For this review, take the finished solid that the model builds, in its own axes (mm). A direction names the side the tool comes from. Coordinates: 2 decimals unless noted, no trailing zeros. Write each loop counter-clockwise with the first axis right and the second up, starting at its lowest first coordinate (ties: lowest second). Pieces come first, ordered by that corner, then holes.
1) We need section B-B on z = -33.25. Write out the cut boundary in (x, y).
2) Insertion check: P1, Ø10, axis at x = 11.5, y = -4.5, coming from the -Z side (3 decimals); P2, Ø10.5, axis at x = 19.5, y = -7.5, coming from the -Z side; P3, Ø6.5, axis at x = 25.84, z = -39.9, coming from the -Y side. Each pin has a flat end and moves straight along its axis. Give the tip position at first contact, or say it passes through.
3) For faces 4 (the face through (30.226, 4.09, -39.007)), 5 (the face through (25, 5.076, -30)), 6 (the face through (31.338, -19, -34)), 7 (the face through (26, -7, -29.903)), 8 (the face through (30.487, -12.894, -27.438)), list the 3-axis set-ups (+Z, -Z, +X, -X, +Y, -Y) from which the entire face can be reached by the end or side of a thin tool; tool diameter is ignored.
4) To check wall thickness, follow line 1 along X through (y, z) = (-13, -28); line 2 along Y through (x, z) = (48.5, -32.5); line 3 along Y through (x, z) = (42, -28.25). State the ranges of each line that lie inside material, in increasing order.
5) We need section D-D on y = 1.75. Write out the cut boundary in (x, z).
6) We need section A-A on x = 44.5. Write out the cut boundary in (y, z).
7) Mouldability with a two-part tool opening along X and no side actions: class faces 1 (the face through (25.911, 4.09, -43.903)), 2 (the face through (49, -8, -34.903)), 3 (the face through (30.487, 1.906, -27.438)) as pulls with the +X half, pulls with the -X half, needs draft (parallel to the pull), parting line crosses it, or undercut.
8) We need section C-C on y = -13.5. Write out the cut boundary in (x, z), then the cut area to 3 significant figures.
Autodesk Inventor part; units mm, degrees
ref_plane "Plano de trabalho1" through (25.8382, -7.4236, -29.9034) normal (0, 0, 1) x (1, 0, 0)
ref_plane "Plano de trabalho2" through (25.638, 5.0764, -94.896) normal (0, -1, 0) x (0, 0, 1)
ref_plane "YZ Plane" through (0, 0, 0) normal (1, 0, 0) x (0, 1, 0)
ref_plane "Plano de trabalho1" through (25.8382, -7.4236, -29.9034) normal (0, 0, 1) x (1, 0, 0)
sketch "Esboço1" plane through (25.8382, -7.4236, -29.9034) normal (0, 0, 1) x (1, 0, 0)
  line L0 (-23, 10.5) -> (23, 10.5)
  line L1 (23, 10.5) -> (23, -10.5)
  line L2 (23, -10.5) -> (-23, -10.5)
  line L3 (-23, -10.5) -> (-23, 10.5)
  line L4 (23, 12.5) -> (-23, 12.5)
  line L5 (-25, 10.5) -> (-25, -10.5)
  line L6 (-23, -12.5) -> (23, -12.5)
  line L7 (25, -10.5) -> (25, 10.5)
  arc A0 (23, -12.5) -> (25, -10.5) centre (23, -10.5) ccw
  arc A1 (-25, -10.5) -> (-23, -12.5) centre (-23, -10.5) ccw
  circle A2 centre (-13, 0) radius 8.5
  circle A3 centre (13, 0) radius 8.5
  line L8 (-23, 10.5) -> (23, -10.5) construction
  line L9 (23, 10.5) -> (-23, -10.5) construction
  line L10 (-3.25, 4.9) -> (3.25, 4.9)
  line L11 (5.25, 6.9) -> (5.25, 7.9)
  line L12 (3.25, 9.9) -> (-3.25, 9.9)
  line L13 (-5.25, 7.9) -> (-5.25, 6.9)
  line L14 (-5.25, 4.9) -> (5.25, 9.9) construction
  line L15 (5.25, 4.9) -> (-5.25, 9.9) construction
  arc A4 (-3.25, 9.9) -> (-5.25, 7.9) centre (-3.25, 7.9) ccw
  arc A5 (-5.25, 6.9) -> (-3.25, 4.9) centre (-3.25, 6.9) ccw
  arc A6 (3.25, 4.9) -> (5.25, 6.9) centre (3.25, 6.9) ccw
  arc A7 (5.25, 7.9) -> (3.25, 9.9) centre (3.25, 7.9) ccw
  line L16 (0, 0) -> (0, -7.4)
  line L17 (-3.25, -9.9) -> (3.25, -9.9)
  line L18 (5.25, -7.9) -> (5.25, -6.9)
  line L19 (3.25, -4.9) -> (-3.25, -4.9)
  line L20 (-5.25, -6.9) -> (-5.25, -7.9)
  line L21 (-5.25, -9.9) -> (5.25, -4.9) construction
  line L22 (5.25, -9.9) -> (-5.25, -4.9) construction
  arc A8 (-3.25, -4.9) -> (-5.25, -6.9) centre (-3.25, -6.9) ccw
  arc A9 (-5.25, -7.9) -> (-3.25, -9.9) centre (-3.25, -7.9) ccw
  arc A10 (3.25, -9.9) -> (5.25, -7.9) centre (3.25, -7.9) ccw
  arc A11 (5.25, -6.9) -> (3.25, -4.9) centre (3.25, -6.9) ccw
  line L23 (-23, 12.5) -> (-25, 12.5)
  line L24 (-25, 12.5) -> (-25, 10.5)
  line L25 (23, 12.5) -> (25, 12.5)
  line L26 (25, 12.5) -> (25, 10.5)
  point P0 (-25.8382, 7.4236)
  dimension "d0" = 2
  dimension "d4" = 46
  dimension "d5" = 21
  dimension "d7" = 17
  dimension "d9" = 17
  dimension "d16" = 7.4
extrude "Extrusão1" add sketch "Esboço1" along normal blind 5 contours L0 L1 L2 L3 | L25 L26 L7 A0 L6 A1 L5 L24 L23 L4
extrude "Extrusão2" add sketch "Esboço1" against normal blind 5 contours L25 L26 L7 A0 L6 A1 L5 L24 L23 L4
sketch "Esboço2" plane through (2.8382, -19.9236, -24.9034) normal (0, -1, 0) x (1, 0, 0)
  line L0 (28.5, -9.5) -> (28.5, -7.75)
  line L1 (28.5, -7.75) -> (17.5, -7.75)
  line L2 (17.5, -7.75) -> (17.5, -9.5)
  line L3 (46, -10) -> (0, -10)
  line L4 (17.5, -10) -> (28.5, -10)
  line L5 (23, -12) -> (31, -12)
  line L6 (23, -12) -> (15, -12)
  line L7 (15, -12) -> (15, -10)
  line L8 (17, -10) -> (15, -10)
  line L9 (31, -12) -> (31, -10)
  line L10 (29, -10) -> (31, -10)
  arc A0 (28.5, -9.5) -> (29, -10) centre (29, -9.5) ccw
  arc A1 (17, -10) -> (17.5, -9.5) centre (17, -9.5) ccw
  point P0 (-2.8382, 24.9034)
  point P1 (23, -10)
  point P2 (17, -10)
  dimension "d24" = 8
  dimension "d25" = 8
  dimension "d26" = 0.5
  dimension "d27" = 0.5
extrude "Extrusão3" cut sketch "Esboço2" against normal up to surface (2 mm away) contours A0 L3 A1 L2 L1 L0
ref_plane "Plano de trabalho2" through (25.638, 5.0764, -94.896) normal (0, -1, 0) x (0, 0, 1)
sketch "Esboço5" plane through (0.8382, 5.0764, -24.9034) normal (0, 1, 0) x (1, 0, 0)
  line L0 (48, 10) -> (2, 10)
  circle A0 centre (25, 15) radius 2
  arc A1 (28.8606, 16.0467) -> (21.1394, 16.0467) centre (25, 15) ccw
  line L1 (19.5, 10) -> (21.1394, 16.0467)
  line L2 (30.5, 10) -> (28.8606, 16.0467)
  line L3 (30.5, 10) -> (19.5, 10)
  line L4 (0, 10) -> (50, 10)
  point P0 (-0.8382, -24.9034)
  dimension "d56" = 4
  dimension "d57" = 2
extrude "Extrusão5" add sketch "Esboço5" against normal blind 2
fillet "Arredondamento3" radius 3 2 edges at (20.3382, 4.0764, -34.9034) (31.3382, 4.0764, -34.9034)
properties part number "suporte ultrasom"
Result:
1. outline: (0.84, -17.92) arc R2 ccw to (2.84, -19.92) - (20.34, -19.92) - (20.34, -17.92) - (2.84, -17.92) - (2.84, 3.08) - (48.84, 3.08) - (48.84, -17.92) - (31.34, -17.92) - (31.34, -19.92) - (48.84, -19.92) arc R2 ccw to (50.84, -17.92) - (50.84, 5.08) - (0.84, 5.08) - close
2. P1: passes through
2. P2: stops at z = -29.9
2. P3: stops at y = 3.08
3. face 4: -Z, +X, +Y, -Y
3. face 5: +Z, -Z, +X, -X, +Y
3. face 6: -Z, -Y
3. face 7: -Z
3. face 8: +Z, -Z
4. line 1: x = 0.84 to 6.42, 19.25 to 21.09, 30.59 to 32.42, 45.25 to 50.84
4. line 2: y = -19.92 to -17.92, 3.08 to 5.08
4. line 3: y = -19.92 to -15.31, 0.47 to 5.08
5. outline: (0.84, -34.9) - (2.84, -34.9) - (2.84, -29.9) - (21.05, -29.9) - (21.05, -24.9) - (0.84, -24.9) - close; (30.63, -29.9) - (48.84, -29.9) - (48.84, -34.9) - (50.84, -34.9) - (50.84, -24.9) - (30.63, -24.9) - close
6. outline: (-19.92, -34.9) - (-17.92, -34.9) - (-17.92, -29.9) - (-13.76, -29.9) - (-13.76, -24.9) - (-19.92, -24.9) - close; (-1.08, -29.9) - (3.08, -29.9) - (3.08, -34.9) - (5.08, -34.9) - (5.08, -24.9) - (-1.08, -24.9) - close
7. face 1: parting line crosses it
7. face 2: needs draft
7. face 3: undercut
8. outline: (0.84, -34.9) - (2.84, -34.9) - (2.84, -29.9) - (6.89, -29.9) - (6.89, -24.9) - (0.84, -24.9) - close; (18.78, -29.9) - (20.77, -29.9) - (20.77, -24.9) - (18.78, -24.9) - close; (30.91, -29.9) - (32.89, -29.9) - (32.89, -24.9) - (30.91, -24.9) - close; (44.78, -29.9) - (48.84, -29.9) - (48.84, -34.9) - (50.84, -34.9) - (50.84, -24.9) - (44.78, -24.9) - close
8. area: 100 mm2
